Geometry check sheet. Reference: the model listing, model coordinates, mm. A direction names the side the tool comes from. Give positions to 0.01 mm unless a question says otherwise; leave off trailing zeros. Write each loop counter-clockwise with the first axis right and the second up, starting at its lowest first coordinate (ties: lowest second). Pieces come first, ordered by that corner, then holes. Notation, with made-up numbers: (32.5, -39) - (71.5, -39) arc R18 ccw to (71.5, -21) - close; hole circle Ø5 at (4, 12.5). An arc over 180 degrees is marked (long way). Use a Markdown table: item, result.
```python
from build123d import *

# Parameters (mm, degrees)
F0_R     = 3.5
F0_R_2   = 3
F1_DEPTH = 25
F2_R     = 8.5
F2_R_2   = 3
F3_DEPTH = 3
F4_R     = 8.5
F4_R_2   = 8
F5_DEPTH = 25


with BuildPart() as f1:
    # F0 (on Front) → F1 (new body)
    with BuildSketch(Plane.XZ):
        Circle(F0_R)
        Circle(F0_R_2, mode=Mode.SUBTRACT)
    extrude(amount=F1_DEPTH)

    # F2 (on Front) → F3 (join)
    with BuildSketch(Plane.XZ):
        Circle(F2_R)
        Circle(F2_R_2, mode=Mode.SUBTRACT)
    extrude(amount=F3_DEPTH)

    # F4 (on face) → F5 (join)
    with BuildSketch(Plane(origin=(0, 0, 0), x_dir=(-1, 0, 0), z_dir=(0, 1, 0))):
        Circle(F4_R)
        Circle(F4_R_2, mode=Mode.SUBTRACT)
    extrude(amount=F5_DEPTH)


solid = f1.part
```
1) Material ranges on L1, parallel to Y at x = 2.25, z = 7.75; L2, parallel to Z at x = 1, y = 10; L3, parallel to X at y = 20, z = 1.5, recorded low to high. Write a range as from..to.
Working result:
| item | result |
|---|---|
| L1 | y = -3..25 |
| L2 | z = -8.44..-7.94, 7.94..8.44 |
| L3 | x = -8.37..-7.86, 7.86..8.37 |
2) Section check D-D on z = 6.5. Record the boundary of the cut face in (x, y), then the cut area to 3 significant figures.
Working result:
| item | result |
|---|---|
| outline | (-5.48, -3) - (5.48, -3) - (5.48, 25) - (4.66, 25) - (4.66, 0) - (-4.66, 0) - (-4.66, 25) - (-5.48, 25) - close |
| area | 73.5 mm² |
3) Depth check by flat-ended pin: P1, Ø2, axis at x = -3.5, z = 3.5, coming from the +Y side; P2, Ø2, axis at x = 3, y = 10.5, coming from the -Z side; P3, Ø5, axis at x = 4, y = 10, coming from the -Z side. Enter the tip coordinate at first touch or a pass-through.
Working result:
| item | result |
|---|---|
| P1 | stops at y = 0 |
| P2 | stops at z = -8.26 |
| P3 | stops at z = -8.37 |
4) Section check C-C on y = 4. Record the boundary of the cut face in (x, z).
Working result:
| item | result |
|---|---|
| outline | circle Ø17 at (0, 0); hole circle Ø16 at (0, 0) |
5) Section check B-B on x = 0. Record the boundary of the cut face in (y, z), then the cut area to 3 significant figures.
Working result:
| item | result |
|---|---|
| outline | (-25, -3.5) - (-3, -3.5) - (-3, -8.5) - (25, -8.5) - (25, -8) - (0, -8) - (0, -3) - (-25, -3) - close; (-25, 3) - (0, 3) - (0, 8) - (25, 8) - (25, 8.5) - (-3, 8.5) - (-3, 3.5) - (-25, 3.5) - close |
| area | 80.0 mm² |
6) Section check A-A on z = 0. Record the boundary of the cut face in (x, y).
Working result:
| item | result |
|---|---|
| outline | (-8.5, -3) - (-3.5, -3) - (-3.5, -25) - (-3, -25) - (-3, 0) - (-8, 0) - (-8, 25) - (-8.5, 25) - close; (3, -25) - (3.5, -25) - (3.5, -3) - (8.5, -3) - (8.5, 25) - (8, 25) - (8, 0) - (3, 0) - close |
7) Mould release check, pull along X, two halves, no side actions. Record for faces 1 (the flat face through (3, -25, 1)), 2 (the cylindrical face through (3.233, -13.846, -1.341)), 3 (the cylindrical face through (1.73, 12.32, -7.81)): pulls with the +X half, pulls with the -X half, needs draft (parallel to the pull), parting line crosses it, or undercut.
Working result:
| item | result |
|---|---|
| face 1 | needs draft |
| face 2 | parting line crosses it |
| face 3 | undercut |
8) Set-up check for faces 4 (the cylindrical face through (-3, -12, 0)), 5 (the flat face through (3.4, 0, 0.1)), 6 (the flat face through (4, -3, 0)): record each of +Z, -Z, +X, -X, +Y, -Y from which the full face is reachable in a straight line by a thin tool's end or side.
Working result:
| item | result |
|---|---|
| face 4 | +Y, -Y |
| face 5 | +Y |
| face 6 | -Y |
